from build123d import *

# Parameters (mm, degrees)
ESQUISSE1_R             = 2.2
BOSS_EXTRU_1_DEPTH      = 5
ESQUISSE3_W             = 5
ESQUISSE3_H             = 5
BOSS_EXTRU_3_DEPTH      = 5
ESQUISSE4_W             = 3
ESQUISSE4_H             = 3
ENL_V_MAT_EXTRU_1_DEPTH = 10


with BuildPart() as part:
    # Esquisse1 → Boss.-Extru.1 (new body)
    with BuildSketch(Plane(origin=(0, 0, 0), x_dir=(0, 0, -1), z_dir=(1, 0, 0))):
        Polygon((-17.5, -40), (-12.5, -40), (-12.5, -35), (-7.5, -35), (-7.5, -40), (-2.5, -40), (-2.5, -35), (2.5, -35), (2.5, -40), (7.5, -40), (7.5, -35), (12.5, -35), (12.5, -40), (17.5, -40), (17.5, 40), (12.5, 40), (12.5, 35), (7.5, 35), (7.5, 40), (2.5, 40), (2.5, 35), (-2.5, 35), (-2.5, 40), (-7.5, 40), (-7.5, 35), (-12.5, 35), (-12.5, 40), (-17.5, 40), align=None)
        with Locations((-7.5, 15)):
            Circle(ESQUISSE1_R, mode=Mode.SUBTRACT)
    extrude(amount=BOSS_EXTRU_1_DEPTH)

    # Esquisse3 → Boss.-Extru.3 (add)
    with BuildSketch(Plane(origin=(0, 40, 0), x_dir=(1, 0, 0), z_dir=(0, 1, 0))):
        with Locations((2.5, -15)):
            Rectangle(ESQUISSE3_W, ESQUISSE3_H)
        with Locations((2.5, -5)):
            Rectangle(ESQUISSE3_W, ESQUISSE3_H)
        with Locations((2.5, 5)):
            Rectangle(ESQUISSE3_W, ESQUISSE3_H)
        with Locations((2.5, 15)):
            Rectangle(ESQUISSE3_W, ESQUISSE3_H)
    extrude(amount=BOSS_EXTRU_3_DEPTH)

    # Esquisse4 → Enlèv. mat.-Extru.1 (cut)
    with BuildSketch(Plane.ZY):
        with Locations((-3, -4.5)):
            Rectangle(ESQUISSE4_W, ESQUISSE4_H)
        with Locations((-9, -4.5)):
            Rectangle(ESQUISSE4_W, ESQUISSE4_H)
        with Locations((3, -4.5)):
            Rectangle(ESQUISSE4_W, ESQUISSE4_H)
        with Locations((9, -4.5)):
            Rectangle(ESQUISSE4_W, ESQUISSE4_H)
        with Locations((9, 4.5)):
            Rectangle(ESQUISSE4_W, ESQUISSE4_H)
        with Locations((3, 4.5)):
            Rectangle(ESQUISSE4_W, ESQUISSE4_H)
        with Locations((-3, 4.5)):
            Rectangle(ESQUISSE4_W, ESQUISSE4_H)
        with Locations((-9, 4.5)):
            Rectangle(ESQUISSE4_W, ESQUISSE4_H)
    extrude(amount=-ENL_V_MAT_EXTRU_1_DEPTH, mode=Mode.SUBTRACT)


solid = part.part
For this review, take the finished solid that the model builds, in its own axes (mm). A direction names the side the tool comes from. Round coordinates to 2 decimals unless told otherwise and drop trailing zeros. Write each loop counter-clockwise with the first axis right and the second up, starting at its lowest first coordinate (ties: lowest second). Pieces come first, ordered by that corner, then holes. Notation, with made-up numbers: (57, -15) - (106, -15) arc R24 ccw to (106, 23) - close; hole circle Ø7 at (80, -33.75). An arc over 180 degrees is marked (long way). Use a Markdown table: item, result.
Q1. We need section C-C (x = 1.5). State how many separate pieces and enclosed holes the cut face has, plus the area to 3 significant figures.
Derived:
| item | result |
|---|---|
| separate pieces | 1 |
| enclosed holes | 9 |
| area | 2,660 mm2 |
Q2. Wall thickness on line 1 along Z through (x, y) = (2.9, 41); line 2 along Y through (x, z) = (2.2, 2); line 3 along Y through (x, z) = (0.6, 12): over which ranges is each line inside the solid? List them lowest first.
Derived:
| item | result |
|---|---|
| line 1 | z = -17.5 to -12.5, -7.5 to -2.5, 2.5 to 7.5, 12.5 to 17.5 |
| line 2 | y = -35 to -6, -3 to 3, 6 to 35 |
| line 3 | y = -35 to 35 |
Q3. Clearance check with flat-ended pins moving along their axes: pin 1 (2.5 mm diameter, centred on x = 2.5, z = -9.5, fed in from -Y); pin 2 (4 mm diameter, centred on y = 30.5, z = -4, fed in from -X). State where each tip first meets the part, or that it passes through.
Derived:
| item | result |
|---|---|
| pin 1 | stops at y = -35 |
| pin 2 | stops at x = 0 |
Q4. We need section A-A (y = 15). Give the boundary of the cut face in (x, z), plus the area to 3 significant figures.
Derived:
| item | result |
|---|---|
| outline | (0, -17.5) - (5, -17.5) - (5, 5.3) - (0, 5.3) - close; (0, 9.7) - (5, 9.7) - (5, 17.5) - (0, 17.5) - close |
| area | 153 mm2 |
Q5. We need section B-B (z = -9.5). Give the boundary of the cut face in (x, y), plus the area to 3 significant figures.
Derived:
| item | result |
|---|---|
| outline | (0, -35) - (5, -35) - (5, -6) - (0, -6) - close; (0, -3) - (5, -3) - (5, 3) - (0, 3) - close; (0, 6) - (5, 6) - (5, 35) - (0, 35) - close |
| area | 320 mm2 |
Q6. Machinability: for faces 1 (the flat face through (2, -35, -10)), 2 (the flat face through (2, 40, 12.5)), 3 (the flat face through (2, -40, -15)), 4 (the flat face through (2, -5, 7.5)), which of the approach directions +Z, -Z, +X, -X, +Y, -Y give a long, thin tool a straight path to every point of the face, cutting with its end or side? Answer none if there is none.
Derived:
| item | result |
|---|---|
| face 1 | +X, -X, -Y |
| face 2 | +X, -X, +Y |
| face 3 | +Z, -Z, +X, -X, -Y |
| face 4 | +X, -X |
Q7. The part is to be moulded in two halves that separate along Y. For faces 5 (the flat face through (2, 45, -5)), 6 (the flat face through (2, -37, -2.5)), 7 (the flat face through (2, -6, -3)), say which applies: pulls with the +Y half, pulls with the -Y half, needs draft (parallel to the pull), parting line crosses it, or undercut.
Derived:
| item | result |
|---|---|
| face 5 | pulls with the +Y half |
| face 6 | needs draft |
| face 7 | undercut |
